Geometry: final body of the model. Coordinates: model frame, mm. A direction names the side the tool comes from. Coordinates: 2 decimals unless noted, no trailing zeros. Loops run counter-clockwise (first coordinate to the right, second up) from the corner with the lowest first, then second, coordinate; pieces in that order, holes last. Notation, with made-up numbers: M -34.75,41 L -23.75,41 A27 ccw -23.75,69 Z; hole C -8,-21 d3. An arc over 180 degrees is marked long. Write each question's results on one line, items separated by ' | '. Start each with the question number.
from build123d import *

# Parameters (mm, degrees)
F2_DEPTH = 50.8


with BuildPart() as f2:
    # F1 (on face) → F2 (new body)
    with BuildSketch(Plane.XZ):
        Polygon((25.4, 25.4), (0, 25.4), (0, 0), (25.4, 0), (25.4, -25.4), (76.2, -25.4), (76.2, 0), (50.8, 0), (50.8, 25.4), (76.2, 25.4), (76.2, 50.8), (25.4, 50.8), align=None)
        Polygon((2.54, 22.86), (27.94, 22.86), (27.94, 48.26), (73.66, 48.26), (73.66, 27.94), (48.26, 27.94), (48.26, -2.54), (73.66, -2.54), (73.66, -22.86), (27.94, -22.86), (27.94, 2.54), (2.54, 2.54), align=None, mode=Mode.SUBTRACT)
    extrude(amount=-F2_DEPTH)


solid = f2.part
Item 1: Section C-C, the plane x = 70. Return loops of the section in (y, z), plus the area to 3 significant figures.
Item 2: Section A-A, the plane x = 5. Return loops of the section in (y, z).
Item 3: Contact query for flat-ended pins moving along their axis: P1, Ø22.5, axis at y = 34.5, z = -12, coming from the -X side; P2, Ø20.5, axis at x = 12, y = 29, coming from the -Z side; P3, Ø15, axis at y = 37, z = 18.5, coming from the -X side; P4, Ø12.5, axis at x = 11.5, y = 24.5, coming from the +Z side. Output: stop coordinate, or through.
Item 4: Pull-direction query (Z, two-part tool) for faces 1 (the flat face through (27.94, 25, 35)), 2 (the flat face through (51, 25, 50.8)), 3 (the flat face through (50, 25, -25.4)); classes: released by +Z, released by -Z, zero draft, split by the parting line, or undercut.
Item 5: Ray query, L1, parallel to Z at x = 57.5, y = 34.5; L2, parallel to Z at x = 15.5, y = 32; L3, parallel to X at y = 43, z = -7. Return the intervals inside material, ascending. Write a range as [from, to].
Item 6: Section D-D, the plane y = 43. Return loops of the section in (x, z).
Item 7: Set-up query: faces 4 (the flat face through (13, 25, 0)), 5 (the flat face through (13, 25, 25.4)), 6 (the flat face through (50.8, 25, 13)), 7 (the flat face through (15, 25, 22.86)). Return all of +Z, -Z, +X, -X, +Y, -Y with unobstructed straight access to the full face (end or side cutting, diameter ignored); none if empty.
Item 8: Section B-B, the plane z = -1. Return loops of the section in (x, y), plus the area to 3 significant figures.
Solutions:
1) outline: M 0,-25.4 L 50.8,-25.4 L 50.8,-22.86 L 0,-22.86 Z; M 0,-2.54 L 50.8,-2.54 L 50.8,0 L 0,0 Z; M 0,25.4 L 50.8,25.4 L 50.8,27.94 L 0,27.94 Z; M 0,48.26 L 50.8,48.26 L 50.8,50.8 L 0,50.8 Z | area: 516 mm²
2) outline: M 0,0 L 50.8,0 L 50.8,2.54 L 0,2.54 Z; M 0,22.86 L 50.8,22.86 L 50.8,25.4 L 0,25.4 Z
3) P1: stops at x = 25.4 | P2: stops at z = 0 | P3: stops at x = 0 | P4: stops at z = 25.4
4) face 1: undercut | face 2: released by +Z | face 3: released by -Z
5) L1: z = [-25.4, -22.86], [-2.54, 0], [25.4, 27.94], [48.26, 50.8] | L2: z = [0, 2.54], [22.86, 25.4] | L3: x = [25.4, 27.94], [73.66, 76.2]
6) outline: M 0,0 L 25.4,0 L 25.4,-25.4 L 76.2,-25.4 L 76.2,0 L 50.8,0 L 50.8,25.4 L 76.2,25.4 L 76.2,50.8 L 25.4,50.8 L 25.4,25.4 L 0,25.4 Z; hole M 2.54,2.54 L 27.94,2.54 L 27.94,-22.86 L 73.66,-22.86 L 73.66,-2.54 L 48.26,-2.54 L 48.26,27.94 L 73.66,27.94 L 73.66,48.26 L 27.94,48.26 L 27.94,22.86 L 2.54,22.86 Z
7) face 4: -Z, -X, +Y, -Y | face 5: +Z, -X, +Y, -Y | face 6: +X, +Y, -Y | face 7: +Y, -Y
8) outline: M 25.4,0 L 27.94,0 L 27.94,50.8 L 25.4,50.8 Z; M 48.26,0 L 76.2,0 L 76.2,50.8 L 48.26,50.8 Z | area: 1,550 mm²
